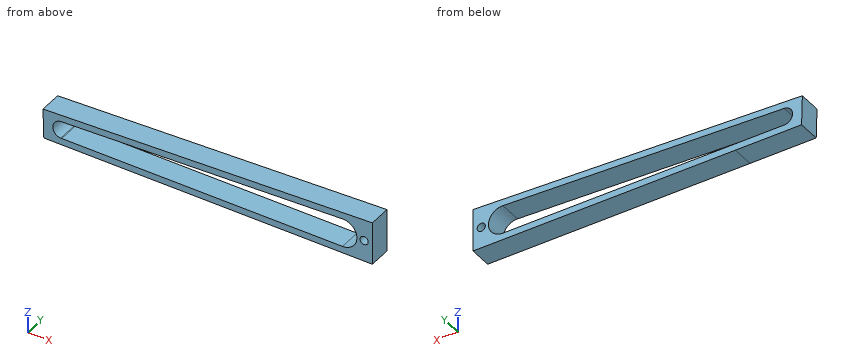
```python
from build123d import *

# Parameters (mm, degrees)
SKETCH1_R           = 2.5
BOSS_EXTRUDE1_DEPTH = 14


with BuildPart() as part:
    # Sketch1 → Boss-Extrude1 (new body)
    with BuildSketch(Plane(origin=(0, 0, 0), x_dir=(1, 0, 0), z_dir=(0, 1, 0))):
        Polygon((-49.807795153, -41.213348306), (-90.005103209, -41.999399148), (-90.480022259, -59.993132832), (109.519977741, -64.056767627), (109.519977741, -38.097723503), align=None)
        with BuildLine():
            Line((-79.112188034, -45.787154937), (91.351489969, -42.453769592))
            ThreePointArc((91.351489969, -42.453769592), (100.137803397, -51.073442227), (91.344504386, -59.685988453))
            Line((91.344504386, -59.685988453), (-79.419326147, -56.217040409))
            ThreePointArc((-79.419326147, -56.217040409), (-84.528615041, -51.150292406), (-79.718159034, -45.799004587))
            ThreePointArc((-79.718159034, -45.799004587), (-79.415345745, -45.784273175), (-79.112188034, -45.787154937))
        make_face(mode=Mode.SUBTRACT)
        with Locations((104.519977741, -51.075218669)):
            Circle(SKETCH1_R, mode=Mode.SUBTRACT)
    extrude(amount=BOSS_EXTRUDE1_DEPTH)


solid = part.part
```
Input: part model. Units: mm. Frame: model coordinates. Coordinates: 2 decimals unless noted, no trailing zeros. Loops run counter-clockwise (first coordinate to the right, second up) from the corner with the lowest first, then second, coordinate; pieces in that order, holes last.
Q1. Section A-A, the plane x = 35.5. Return the cut outline in (y, z), and give its area (3 significant figures).
Results are:
outline: (0, 39.55) - (14, 39.55) - (14, 43.55) - (0, 43.55) - close; (0, 58.55) - (14, 58.55) - (14, 62.55) - (0, 62.55) - close
area: 112 mm2
Q2. Section C-C, the plane x = 89. Return the cut outline in (y, z).
Results are:
outline: (0, 38.5) - (14, 38.5) - (14, 42.5) - (0, 42.5) - close; (0, 59.64) - (14, 59.64) - (14, 63.64) - (0, 63.64) - close
Q3. Section B-B, the plane y = 5.25. Return the cut outline in (x, z), and give its area (3 significant figures).
Results are:
outline: (-90.48, 59.99) - (-90.01, 42) - (109.52, 38.1) - (109.52, 64.06) - close; hole (-79.42, 56.22) arc R5.22 ccw (long way) to (-79.11, 45.79) - (91.35, 42.45) arc R8.62 ccw (long way) to (91.34, 59.69) - close; hole circle Ø5 at (104.52, 51.08)
area: 1,850 mm2
Q4. Contact query for flat-ended pins moving along their axis: pin 1 (2 mm diameter, centred on x = -2.5, z = 55.5, fed in from +Y); pin 2 (6 mm diameter, centred on x = -61.5, y = 6, fed in from +Z); pin 3 (1 mm diameter, centred on x = 23.5, y = 6, fed in from +Z); pin 4 (6 mm diameter, centred on y = 2, z = 42.5, fed in from -X). Output: stop coordinate, or through.
Results are:
pin 1: passes through
pin 2: stops at z = 60.64
pin 3: stops at z = 62.32
pin 4: stops at x = -90.1
Q5. Line query: line 1 along X through (y, z) = (3.25, 51); line 2 along X through (y, z) = (4.5, 55.5); line 3 along Z through (x, y) = (39, 4.5). Output: solid intervals per line, ascending.
Results are:
line 1: x = -90.24 to -84.53, 100.14 to 102.02, 107.02 to 109.52
line 2: x = -90.36 to -81.95, 98.91 to 109.52
line 3: z = 39.48 to 43.48, 58.62 to 62.62
